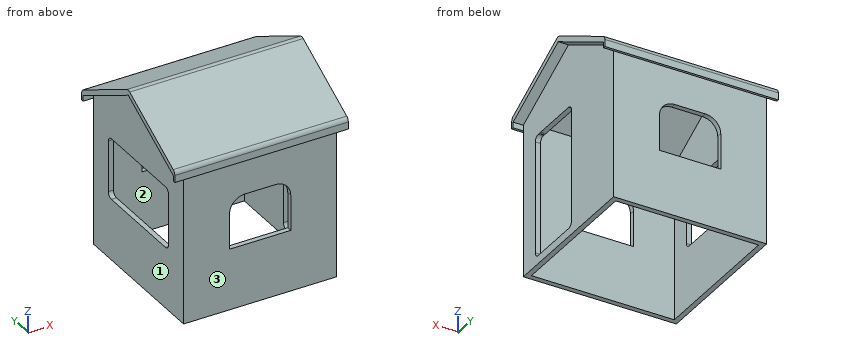
Autodesk Inventor part; units mm, degrees
ref_plane "Plano de trabajo1" through (75, 0, 0) normal (1, 0, 0) x (0, 0, -1)
ref_plane "Plano de trabajo2" through (150, 25, 68) normal (0, 0, 1) x (1, 0, 0)
ref_plane "YZ Plane" through (0, 0, 0) normal (1, 0, 0) x (0, 1, 0)
sketch "Boceto1" plane through (0, 0, 0) normal (0, 0, 1) x (1, 0, 0)
  line L0 (0, 0) -> (150, 0)
  line L1 (150, 0) -> (150, 150)
  line L2 (150, 150) -> (0, 150)
  line L3 (0, 150) -> (0, 0)
  line L4 (5, 145) -> (145, 145)
  line L5 (145, 145) -> (145, 5)
  line L6 (145, 5) -> (5, 5)
  line L7 (5, 5) -> (5, 145)
  dimension "d0" = 150
  dimension "d1" = 150
  dimension "d2" = 5
extrude "Extrusión1" add sketch "Boceto1" along normal blind 150
sketch "Boceto2" plane through (150, 0, 0) normal (1, 0, 0) x (0, 0, -1)
  line L0 (-150, 0) -> (-150, 150)
  line L1 (-150, 75) -> (-190, 75) construction
  line L2 (-190, 75) -> (-150, 150)
  line L3 (0, 0) -> (-150, 0) construction
  line L4 (-150, 0) -> (-190, 75)
  dimension "d5" = 40
extrude "Extrusión2" add sketch "Boceto2" against normal blind 5
ref_plane "Plano de trabajo1" through (75, 0, 0) normal (1, 0, 0) x (0, 0, -1)
mirror "Simetría1" about plane through (75, 0, 0) normal (1, 0, 0) of "Extrusión2"
sketch "Boceto3" plane through (0, 150, 0) normal (0, 1, 0) x (1, 0, 0)
  line L0 (105, -60) -> (45, -60)
  line L1 (45, -60) -> (45, -95)
  line L2 (60, -110) -> (90, -110)
  line L3 (105, -95) -> (105, -60)
  line L4 (150, 0) -> (0, 0)
  line L5 (145, -150) -> (5, -150)
  arc A0 (90, -110) -> (105, -95) centre (90, -95) ccw
  arc A1 (45, -95) -> (60, -110) centre (60, -95) ccw
  point P0 (45, -110)
  point P1 (105, -110)
  point P2 (75, -60)
  point P3 (75, 0)
  dimension "d8" = 60
  dimension "d9" = 50
  dimension "d10" = 40
  dimension "d11" = 15
extrude "Extrusión3" cut sketch "Boceto3" against normal through all
sketch "Boceto4" plane through (150, 0, 0) normal (1, 0, 0) x (0, 0, -1)
  line L0 (-13, 20) -> (-123, 20)
  line L1 (-128, 25) -> (-128, 75)
  line L2 (-123, 80) -> (-13, 80)
  line L3 (-8, 75) -> (-8, 25)
  line L4 (0, 0) -> (0, 150)
  line L5 (0, 0) -> (-150, 0)
  arc A0 (-123, 80) -> (-128, 75) centre (-123, 75) ccw
  arc A1 (-8, 75) -> (-13, 80) centre (-13, 75) ccw
  arc A2 (-13, 20) -> (-8, 25) centre (-13, 25) ccw
  arc A3 (-128, 25) -> (-123, 20) centre (-123, 25) ccw
  point P0 (-128, 80)
  point P1 (-128, 20)
  point P2 (-8, 80)
  dimension "d14" = 120
  dimension "d15" = 60
  dimension "d16" = 8
  dimension "d17" = 20
  dimension "d18" = 5
extrude "Extrusión4" cut sketch "Boceto4" against normal up to surface (5 mm away)
sketch "Boceto5" plane through (0, 0, 0) normal (-1, 0, 0) x (0, 0, 1)
  line L0 (65, 125) -> (115, 125)
  line L1 (120, 120) -> (120, 30)
  line L2 (115, 25) -> (65, 25)
  line L3 (60, 30) -> (60, 120)
  line L4 (0, 150) -> (0, 0)
  arc A0 (120, 120) -> (115, 125) centre (115, 120) ccw
  arc A1 (115, 25) -> (120, 30) centre (115, 30) ccw
  arc A2 (65, 125) -> (60, 120) centre (65, 120) ccw
  arc A3 (60, 30) -> (65, 25) centre (65, 30) ccw
  point P0 (60, 150)
  point P1 (120, 25)
  point P2 (120, 125)
  point P3 (60, 25)
  point P4 (60, 75)
  point P5 (0, 75)
  dimension "d21" = 60
  dimension "d22" = 100
  dimension "d23" = 60
  dimension "d24" = 5
extrude "Extrusión5" cut sketch "Boceto5" against normal blind 10
sketch "Boceto6" plane through (150, 0, 0) normal (1, 0, 0) x (0, 0, -1)
  line L0 (-190, 75) -> (-150, 0)
  line L1 (-150, 150) -> (-190, 75)
  line L2 (-154.4118, 152.3529) -> (-195.6667, 75)
  line L3 (-195.6667, 75) -> (-154.4118, -2.3529)
  line L4 (-154.4118, 152.3529) -> (-144.4118, 152.3529)
  line L5 (-144.4118, 152.3529) -> (-144.4118, 150)
  line L6 (-154.4118, -2.3529) -> (-144.4118, -2.3529)
  line L7 (-144.4118, -2.3529) -> (-144.4118, 0)
  line L8 (0, 0) -> (-150, 0)
  line L9 (0, 150) -> (-150, 150)
  dimension "d27" = 5
  dimension "d28" = 10
extrude "Extrusión6" add sketch "Boceto6" along normal blind 10 and the other way blind 160
fillet "Empalme1" radius 5 3 edges at (75, 152.3529, 154.4118) (75, 75, 195.6667) (75, -2.3529, 154.4118)
sketch "Boceto7" plane through (150, 25, 8) normal (0, 0, 1) x (1, 0, 0)
  circle A0 centre (-2.5, 2.5) radius 1.25
  line L0 (0, 50) -> (0, 0)
  line L1 (0, 0) -> (-5, 0)
  point P0 (-150, -25)
  point P1 (-2.5, 0)
  dimension "d34" = 2.5
  dimension "d35" = 2.5
  dimension "d36" = 2.5
extrude "Extrusión7" cut sketch "Boceto7" against normal blind 3
ref_plane "Plano de trabajo2" through (150, 25, 68) normal (0, 0, 1) x (1, 0, 0)
mirror "Simetría2" about plane through (150, 25, 68) normal (0, 0, 1) of "Extrusión7"
properties part number "CasaJugueteAPM" material "Plástico ABS"
The listing builds one solid part. Answer for the finished solid, in the listing's coordinates (mm). Face numbers are marked on the shaded views. A direction names the side the tool comes from. Give positions to 0.01 mm unless a question says otherwise; leave off trailing zeros. Write each loop counter-clockwise with the first axis right and the second up, starting at its lowest first coordinate (ties: lowest second). Pieces come first, ordered by that corner, then holes.
1) Section B-B (y = 48) is taken. Write down the section's boundary in (x, z), and give its area (3 significant figures).
2) Given P1, Ø5, axis at x = 13.5, z = 170.5, coming from the +Y side; P2, Ø3, axis at x = 127.5, y = 54, coming from the +Z side; P3, Ø5, axis at x = 113.5, y = 24, coming from the +Z side, each flat-ended and moving along its own axis, determine where each tip first touches the part or whether it passes through.
3) Section C-C (z = 27) is taken. Write down the section's boundary in (x, y).
4) A tool of negligible diameter and unlimited length cuts with its end or side. For the marked faces 1, 2 and 3, from which of +Z, -Z, +X, -X, +Y, -Y can it reach the whole face along a straight path? Write none if from no direction.
5) Find the intervals of material crossed by L1, parallel to Y at x = 147.5, z = 130.15; L2, parallel to Y at x = 140.5, z = 69, in increasing order.
6) Section D-D (x = 14.5) is taken. Write down the section's boundary in (y, z).
7) Section A-A (x = 99) is taken. Write down the section's boundary in (y, z), and give its area (3 significant figures).
Response:
1. outline: (-10, 175.6) - (0, 175.6) - (0, 120) - (5, 120) - (5, 175.6) - (145, 175.6) - (145, 128) - (150, 128) - (150, 175.6) - (160, 175.6) - (160, 181.27) - (-10, 181.27) - close; (0, 0) - (5, 0) - (5, 60) - (0, 60) - close; (145, 0) - (150, 0) - (150, 8) - (145, 8) - close
1. area: 1,820 mm2
2. P1: stops at y = 126.88
2. P2: stops at z = 185.27
2. P3: stops at z = 169.8
3. outline: (0, 0) - (150, 0) - (150, 20) - (145, 20) - (145, 5) - (5, 5) - (5, 145) - (145, 145) - (145, 80) - (150, 80) - (150, 150) - (0, 150) - close
4. face 1: -Z, -X
4. face 2: -Z
4. face 3: -Z, +X, -X, -Y
5. L1: y = 0 to 26.25, 28.75 to 150
5. L2: y = 0 to 5, 145 to 150
6. outline: (-2.35, 144.41) - (0, 144.41) - (0, 0) - (5, 0) - (5, 150) - (0, 150) - (75, 190) - (150, 150) - (145, 150) - (145, 0) - (150, 0) - (150, 144.41) - (152.35, 144.41) - (152.35, 151.41) arc R5 ccw to (149.71, 155.82) - (77.35, 194.41) arc R5 ccw to (72.65, 194.41) - (0.29, 155.82) arc R5 ccw to (-2.35, 151.41) - close
7. outline: (-2.35, 144.41) - (0, 144.41) - (0, 107) - (5, 107) - (5, 150) - (0, 150) - (75, 190) - (150, 150) - (145, 150) - (145, 107) - (150, 107) - (150, 144.41) - (152.35, 144.41) - (152.35, 151.41) arc R5 ccw to (149.71, 155.82) - (77.35, 194.41) arc R5 ccw to (72.65, 194.41) - (0.29, 155.82) arc R5 ccw to (-2.35, 151.41) - close; (0, 0) - (5, 0) - (5, 60) - (0, 60) - close; (145, 0) - (150, 0) - (150, 60) - (145, 60) - close
7. area: 1,930 mm2
